Part model, mm, in its own coordinate system. Round coordinates to 2 decimals unless told otherwise and drop trailing zeros. Write each loop counter-clockwise with the first axis right and the second up, starting at its lowest first coordinate (ties: lowest second). Pieces come first, ordered by that corner, then holes. Notation, with made-up numbers: M -2.75,73 L 22.25,73 A26 ccw 22.25,101 Z; hole C 12.25,77 d1. An arc over 180 degrees is marked long. Use a Markdown table: item, result. Add a question column.
1) Slice it at C-C on y = 57.5. Write the cut outline in (x, z).
2) Slice it at A-A on z = 39.65. Write the cut outline in (x, y), plus the area to 3 significant figures.
3) Slice it at B-B on x = 38. Write the cut outline in (y, z), plus the area to 3 significant figures.
4) Wall check: probe 1 along X at (y, z) = (95, 39.75); probe 2 along X at (y, z) = (65, 38.15); probe 3 along Y at (x, z) = (6, 38.75). Give the ranges that are in metal, low to high.
Autodesk Inventor part; units mm, degrees
ref_plane "Plano de trabajo14" through (0, 0, 40) normal (0, 0, 1) x (1, 0, 0)
ref_plane "Plano de trabajo15" through (0, 0, 40) normal (0, 0, -1) x (-1, 0, 0)
ref_plane "YZ Plane" through (0, 0, 0) normal (1, 0, 0) x (0, 1, 0)
ref_plane "Plano de trabajo14" through (0, 0, 40) normal (0, 0, 1) x (1, 0, 0)
ref_plane "Plano de trabajo15" through (0, 0, 40) normal (0, 0, -1) x (-1, 0, 0)
sketch "Boceto24" plane through (0, 0, 40) normal (0, 0, -1) x (-1, 0, 0)
  arc A0 (0, 95) -> (-5, 100) centre (-5, 95) ccw
  arc A1 (-30, 100) -> (-35, 95) centre (-30, 95) ccw
  arc A2 (-5, 100) -> (-30, 100) centre (-17.5, 41.3165) ccw
  arc A3 (-10, 75) -> (0, 95) centre (-34.6648, 99.8324) ccw
  line L0 (-47.9872, 67.409) -> (-27.7264, 51.2004)
  arc A4 (-27.7264, 51.2004) -> (-23.2542, 52.043) centre (-25.8523, 53.543) ccw
  arc A5 (-48.7112, 71.2516) -> (-47.9872, 67.409) centre (-46.1131, 69.7516) ccw
  arc A6 (-35, 95) -> (-48.7112, 71.2516) centre (61.3869, 23.5187) ccw
  arc A7 (-10, 75) -> (-23.2542, 52.043) centre (86.6601, 3.8886) ccw
  point P0 (0, 0)
  point P1 (0, 100)
  point P2 (-35, 100)
  point P3 (-25, 49.0192)
  point P4 (-50, 69.0192)
extrude "Extrusión16" add sketch "Boceto24" along normal blind 2
sketch "Boceto34" plane through (0, 0, 40) normal (0, 0, 1) x (1, 0, 0)
  line L0 (30.8918, 53.7327) -> (44.3961, 64.5361)
  line L1 (37.8568, 59.3047) -> (40.3278, 59.3047) construction
  line L2 (30.466, 53.3921) -> (44.3961, 64.5361)
  line L3 (30.466, 53.3921) -> (37.431, 58.9641)
  line L4 (37.431, 58.9641) -> (39.902, 58.9641) construction
  arc A0 (44.3961, 64.5361) -> (30.466, 53.3921) centre (38.9746, 57.0346) ccw
  point P0 (0, 0)
extrude "Extrusión26" cut sketch "Boceto34" against normal blind 10
equation "\"Radio_pliegue\" = Grosor"
equation "\"Anchura_desahogo_plegado\" = Grosor"
equation "\"Profundidad_desahogo_plegado\" = 0.5 * Grosor"
equation "\"Tamaño_destalonado\" = 4 * Grosor"
equation "\"Remanente_mínimo\" = 2 * Grosor"
equation "\"Radiodetransición\" = Radio_pliegue"
equation "\"Tamaño_de_radio_de_Jacobi\" = Radio_pliegue"
equation "\"TamañoSeparación\" = Grosor"
properties part number "brazocuadrado"
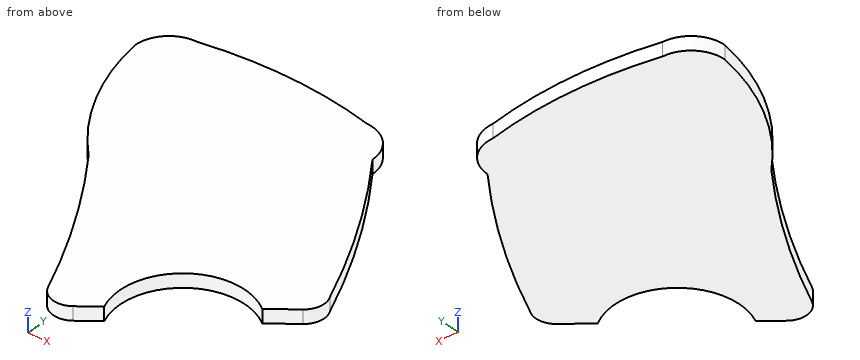
Entries:
| question | item | result |
|---|---|---|
| 1 | outline | M 20.7,38 L 29.73,38 L 29.73,40 L 20.7,40 Z |
| 2 | outline | M 0,95 A35 ccw 10,75 A120 cw 23.25,52.04 A3 ccw 27.73,51.2 L 30.47,53.39 A9.26 cw 44.4,64.54 L 47.99,67.41 A3 ccw 48.71,71.25 A120 ccw 35,95 A5 ccw 30,100 A60 ccw 5,100 A5 ccw Z |
| 2 | area | 1,420 mm^2 |
| 3 | outline | M 66.24,38 L 90.77,38 L 90.77,40 L 66.24,40 Z |
| 3 | area | 49.1 mm^2 |
| 4 | probe 1 | x = 0 to 35 |
| 4 | probe 2 | x = 16.61 to 34.26, 43.69 to 44.98 |
| 4 | probe 3 | y = 79.75 to 100.2 |
